Answer from the drawing. Dimensions are ordinates in mm from the lowest x, y and z of the part. A direction names the side the tool comes from. Give positions to 0.01 mm unless a question says otherwise; leave off trailing zeros. Order: outer loops, then holes, each group sorted by start corner. A loop starts at its lowest first (then second) coordinate and runs counter-clockwise, first axis right, second up.
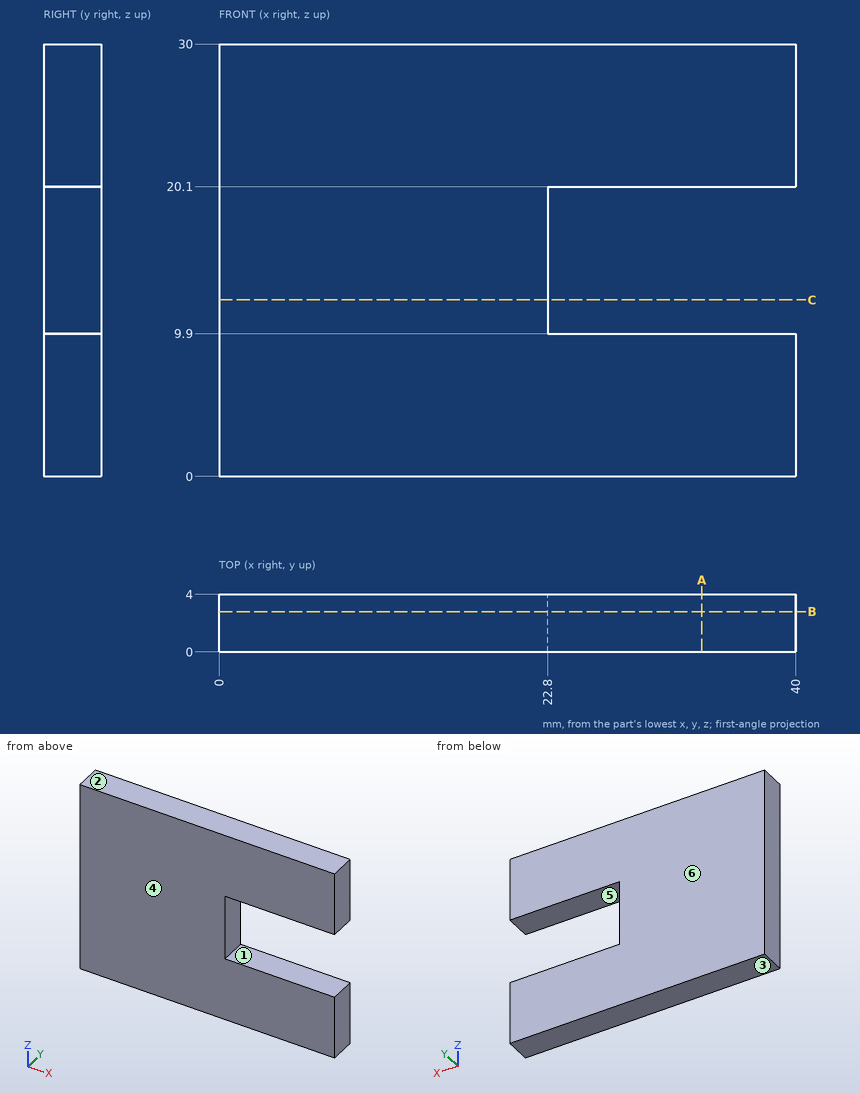
1. Which of the six approach directions +Z, -Z, +X, -X, +Y, -Y give full straight-line access (tool end or side, diameter ignored) to the marked faces 5 and 6?
Findings below:
face 5: +X, +Y, -Y
face 6: +Z, -Z, +X, -X, +Y
2. The part is cut by section B-B (y = 2.8). Write down the section's boundary in (x, z), then the cut area to 3 significant figures.
Findings below:
outline: (0, 0) - (40, 0) - (40, 9.9) - (22.8, 9.9) - (22.8, 20.1) - (40, 20.1) - (40, 30) - (0, 30) - close
area: 1,020 mm2
3. The part is cut by section C-C (z = 12.25). Write down the section's boundary in (x, y).
Findings below:
outline: (0, 0) - (22.8, 0) - (22.8, 4) - (0, 4) - close
4. Straight lines are drawn through the part: probe 1 along Z at (x, y) = (30, 2.45); probe 2 along X at (y, z) = (3.6, 18.25). For each, find the intervals that lie inside material, in ascending order.
Findings below:
probe 1: z = 0 to 9.9, 20.1 to 30
probe 2: x = 0 to 22.8
5. The part is cut by section A-A (x = 33.5). Write down the section's boundary in (y, z).
Findings below:
outline: (0, 0) - (4, 0) - (4, 9.9) - (0, 9.9) - close; (0, 20.1) - (4, 20.1) - (4, 30) - (0, 30) - close
6. The mould has two halves that part along Z. Classify the marked faces 1, 2, 3 and 4: pulls with the +Z half, pulls with the -Z half, needs draft (parallel to the pull), parting line crosses it, or undercut.
Findings below:
face 1: undercut
face 2: pulls with the +Z half
face 3: pulls with the -Z half
face 4: needs draft
